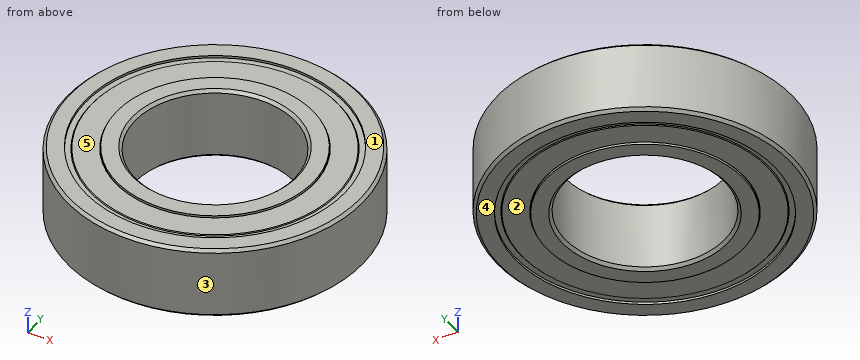
from build123d import *


with BuildPart() as part:
    # Sketch → Revolution (revolve)
    with BuildSketch(Plane.XZ):
        Polygon((-18.5, 4.146447), (-18.5, -4.146447), (-18.146447, -4.5), (-16.2, -4.5), (-16.2, -4.2), (-15.5, -4.2), (-15.4, -4.3), (-12.4, -4.3), (-12.3, -4.2), (-12.3, -4.5), (-10.353553, -4.5), (-10, -4.146447), (-10, 4.146447), (-10.353553, 4.5), (-12.3, 4.5), (-12.3, 4.2), (-12.4, 4.3), (-15.4, 4.3), (-15.5, 4.2), (-16.2, 4.2), (-16.2, 4.5), (-18.146447, 4.5), align=None)
    revolve(axis=Axis((0, 0, 0), (0, 0, 1)))


solid = part.part
Here's how the part is built. I have some questions about the finished solid (model axes, mm). Face numbers are marked on the shaded views. A direction names the side the tool comes from. Round coordinates to 2 decimals unless told otherwise and drop trailing zeros. Write each loop counter-clockwise with the first axis right and the second up, starting at its lowest first coordinate (ties: lowest second). Pieces come first, ordered by that corner, then holes. Notation, with made-up numbers: (-16, 62.5) -> (14, 62.5) arc R18 ccw to (14, 92.5) -> close; hole circle Ø10 at (-14, -20.5). An arc over 180 degrees is marked (long way). One line per item, written item: value.
1) If I drill on line 1 (X direction, y = 0, z = -1.5); line 2 (X direction, y = 0, z = 4.4), over which ranges is the centre line in solid material (lowest first)? Write a range as [from, to].
Filled sheet:
line 1: x = [-18.5, -10], [10, 18.5]
line 2: x = [-18.25, -16.2], [-12.3, -10.25], [10.25, 12.3], [16.2, 18.25]
2) Suppose I cut it at A-A on z = -1.75. List the corners of the cut face in (x, y) for me, plus the area to 3 significant figures.
Filled sheet:
outline: circle Ø37 at (0, 0); hole circle Ø20 at (0, 0)
area: 761 mm2
3) We'd pull the mould along Y, two halves only. Please class the marked faces 3, 4 and 5: released by +Y, released by -Y, zero draft, split by the parting line, or undercut.
Filled sheet:
face 3: split by the parting line
face 4: zero draft
face 5: undercut
4) For the marked faces 1 and 2, which set-ups out of +Z, -Z, +X, -X, +Y, -Y let a thin tool reach every point of the face, with its end or its side?
Filled sheet:
face 1: +Z, +X, -X, +Y, -Y
face 2: -Z
5) I'm going to push flat-ended pins straight in: pin 1 Ø1.5 at (x, z) = (12, -1) entering from +Y; pin 2 Ø1 at (y, z) = (9.5, 0) entering from -X; pin 3 Ø5 at (x, z) = (-3.5, 2) entering from -Y. Where does each tip first touch, or does it pass through?
Filled sheet:
pin 1: stops at y = 14.69
pin 2: stops at x = -16.16
pin 3: stops at y = -18.47
